Design review of the part built by this model. Coordinates are the model's own, in mm. A direction names the side the tool comes from. Give positions to 0.01 mm unless a question says otherwise; leave off trailing zeros. Order: outer loops, then holes, each group sorted by start corner. A loop starts at its lowest first (then second) coordinate and runs counter-clockwise, first axis right, second up. Notation, with made-up numbers: M -36,-10 L -2,-10 A21 cw -2,12 Z; hole C -5,0 d9. An arc over 180 degrees is marked long. Answer as a JSON object with one key per item and string values.
from build123d import *

# Parameters (mm, degrees)
SKETCH2_W           = 120
SKETCH2_H           = 150
BOSS_EXTRUDE1_DEPTH = 10
SKETCH3_R           = 30
CUT_EXTRUDE1_DEPTH  = 5
SKETCH4_R           = 22.5
CUT_EXTRUDE2_DEPTH  = 5
FILLET1_SIZE        = 30
FILLET1_SIZE_2      = 10


with BuildPart() as part:
    # Sketch2 → Boss-Extrude1 (new body)
    with BuildSketch(Plane(origin=(0, 0, 0), x_dir=(1, 0, 0), z_dir=(0, 1, 0))):
        Rectangle(SKETCH2_W, SKETCH2_H)
    extrude(amount=BOSS_EXTRUDE1_DEPTH)

    # Sketch3 → Cut-Extrude1 (cut)
    with BuildSketch(Plane(origin=(0, 10, 0), x_dir=(1, 0, 0), z_dir=(0, 1, 0))):
        with Locations((35, 0)):
            Circle(SKETCH3_R)
        with Locations((-35, 0)):
            Circle(SKETCH3_R)
    extrude(amount=-CUT_EXTRUDE1_DEPTH, mode=Mode.SUBTRACT)

    # Sketch4 → Cut-Extrude2 (cut)
    with BuildSketch(Plane(origin=(0, 5, 0), x_dir=(1, 0, 0), z_dir=(0, 1, 0))):
        with Locations(Location((-35, 0, 0), (0, 0, 270))):
            Circle(SKETCH4_R)
        with Locations(Location((35, 0, 0), (0, 0, 270))):
            Circle(SKETCH4_R)
    extrude(amount=-CUT_EXTRUDE2_DEPTH, mode=Mode.SUBTRACT)

    # Fillet1
    # an asymmetric fillet: 30, 10 mm, written as the material it takes off along each edge
    with BuildSketch(Plane(origin=(135, 0, -75), x_dir=(0, 0, 1), z_dir=(-1, 0, 0))) as fillet1_piece_1:
        with BuildLine():
            Bezier((FILLET1_SIZE, 0), (0, 0), (0, FILLET1_SIZE_2), weights=[1, 0.707106781, 1])
            Line((0, FILLET1_SIZE_2), (0, 0))
            Line((0, 0), (FILLET1_SIZE, 0))
        make_face()
    extrude(amount=270, mode=Mode.SUBTRACT)
    with BuildSketch(Plane(origin=(-135, 0, 75), x_dir=(0, 1, 0), z_dir=(1, 0, 0))) as fillet1_piece_2:
        with BuildLine():
            Bezier((FILLET1_SIZE_2, 0), (0, 0), (0, -FILLET1_SIZE), weights=[1, 0.707106781, 1])
            Line((0, -FILLET1_SIZE), (0, 0))
            Line((0, 0), (FILLET1_SIZE_2, 0))
        make_face()
    extrude(amount=270, mode=Mode.SUBTRACT)


solid = part.part
(1) Tool access review of faces 5 (the cylindrical face through (-5.02, 7.54, 1.07)), 6 (the cylindrical face through (-56.965, 2.535, -4.878)): name each direction out of +Z, -Z, +X, -X, +Y, -Y from which nothing blocks a thin tool from reaching the whole face with its end or side.
Checked values:
{"face 5": "+Y", "face 6": "+Y, -Y"}
(2) We need section A-A (z = 0). Write out the cut boundary in (x, y), plus the area to 3 significant figures.
Checked values:
{"outline": "M -60,0 L -57.5,0 L -57.5,5 L -60,5 Z; M -12.5,0 L 12.5,0 L 12.5,5 L 5,5 L 5,10 L -5,10 L -5,5 L -12.5,5 Z; M 57.5,0 L 60,0 L 60,5 L 57.5,5 Z", "area": "200 mm^2"}
(3) Draft analysis for pull direction X (two halves, no side actions). For faces 1 (the cylindrical face through (13.035, 2.535, -4.878)), 2 (the flat face through (-1, 10, -1)), 3 (the flat face through (60, 4, 1)), 4 (the flat face through (-60, 4, 1)), state which applies: +X half, -X half, draft (parallel to the pull), parting line (faces both ways), or undercut.
Checked values:
{"face 1": "undercut", "face 2": "draft", "face 3": "+X half", "face 4": "-X half"}
(4) Insertion check: pin 1 (2 mm diameter, centred on x = -18.5, y = 6.5, fed in from -Z); pin 2 (3 mm diameter, centred on x = -3.5, y = 9, fed in from +Z); pin 3 (6 mm diameter, centred on x = -31, y = 1, fed in from -Z). Each pin has a flat end and moves straight along its axis. Give the tip position at first contact, or say it passes through.
Checked values:
{"pin 1": "stops at z = -74.05", "pin 2": "stops at z = 75", "pin 3": "stops at z = -69"}
(5) To check wall thickness, follow L1, parallel to X at y = 8.5, z = 24; L2, parallel to X at y = 3.85, z = 0; L3, parallel to X at y = 6.2, z = 0. State the ranges of each line that lie inside material, in increasing order. Write a range as from..to.
Checked values:
{"L1": "x = -60..-53, -17..17, 53..60", "L2": "x = -60..-57.5, -12.5..12.5, 57.5..60", "L3": "x = -5..5"}
